from build123d import *

# Parameters (mm, degrees)
SKETCH_1_W           = 33.2
SKETCH_1_H           = 22
SKETCH_1_R           = 1.6
EXTRUDE_1_DEPTH      = 7
SKETCH_2_W           = 33.2
SKETCH_2_H           = 10.5
EXTRUDE_2_DEPTH      = 2
EXTRUDE_3_DEPTH      = 60
SKETCH_4_W           = 2
SKETCH_4_H           = 10.5
EXTRUDE_4_DEPTH      = 38.5
SKETCH_5_W           = 4
SKETCH_5_H           = 10.5
EXTRUDE_5_DEPTH      = 2
SKETCH_6_W           = 4
SKETCH_6_H           = 10.5
EXTRUDE_6_DEPTH      = 19.5
SKETCH_7_W           = 6
SKETCH_7_H           = 93.2
EXTRUDE_7_DEPTH      = 2
SKETCH_8_W           = 93.2
SKETCH_8_H           = 5
EXTRUDE_8_DEPTH      = 3
SKETCH_10_W          = 93.2
SKETCH_10_H          = 2
EXTRUDE_9_DEPTH      = 5.5
SKETCH_12_W          = 18
SKETCH_12_H          = 2
CUT_EXTRUDE_1_DEPTH  = 5.5
SKETCH_13_W          = 40
SKETCH_13_H          = 5
EXTRUDE_10_DEPTH     = 3.5
CUT_EXTRUDE_2_REACH  = 70.879
SKETCH_15_W          = 15.5
SKETCH_15_H          = 5
SKETCH_16_W          = 3.5
SKETCH_16_H          = 2.5
EXTRUDE_12_DEPTH     = 2
CUT_EXTRUDE_3_REACH  = 71.313
CHAMFER_1_SIZE       = 3.5
SKETCH_18_R          = 1.65
EXTRUDE_13_DEPTH     = 2
FILLET_1_R           = 2
SKETCH_19_W          = 4.5
SKETCH_19_H          = 21.5
CUT_EXTRUDE_4_DEPTH  = 5
CHAMFER_2_SIZE       = 3
CUT_EXTRUDE_5_REACH  = 74.561
SKETCH_20_R          = 1.65
EXTRUDE_14_REACH     = 73.895
SKETCH_21_R          = 4.5
SKETCH_21_R_2        = 1.65
EXTRUDE_15_DEPTH     = 6
EXTRUDE_16_DEPTH     = 4
CUT_EXTRUDE_6_REACH  = 83.84
SKETCH_24_R          = 1.65
CUT_EXTRUDE_7_REACH  = 84.171
SKETCH_26_W          = 2
SKETCH_26_H          = 10.5
CUT_EXTRUDE_8_DEPTH  = 5
SKETCH_27_W          = 2
SKETCH_27_H          = 2
EXTRUDE_17_DEPTH     = 10
CUT_EXTRUDE_9_DEPTH  = 2
CUT_EXTRUDE_10_REACH = 84.426
SKETCH_29_R          = 5.5
SKETCH_30_W          = 63
SKETCH_30_H          = 2
EXTRUDE_18_DEPTH     = 1


with BuildPart() as part:
    # 草图1 → 凸台-拉伸1 (new body)
    with BuildSketch(Plane(origin=(0, 0, 0), x_dir=(0, 0, -1), z_dir=(1, 0, 0))):
        with Locations((12.6, -4.5)):
            Rectangle(SKETCH_1_W, SKETCH_1_H)
        Circle(SKETCH_1_R, mode=Mode.SUBTRACT)
        with Locations((20, 0)):
            Circle(SKETCH_1_R, mode=Mode.SUBTRACT)
    extrude(amount=EXTRUDE_1_DEPTH)

    # 草图2 → 凸台-拉伸2 (add)
    with BuildSketch(Plane(origin=(7, 0, 0), x_dir=(0, 0, -1), z_dir=(1, 0, 0))):
        with Locations((12.6, 11.75)):
            Rectangle(SKETCH_2_W, SKETCH_2_H)
    extrude(amount=-EXTRUDE_2_DEPTH)

    # 草图3 → 凸台-拉伸3 (add)
    with BuildSketch(Plane.XY.offset(4)):
        Polygon((7, -15.5), (1, -15.5), (1, 4.5), (3, 4.5), (3, 6.5), (7, 6.5), align=None)
    extrude(amount=EXTRUDE_3_DEPTH)

    # 草图4 → 凸台-拉伸4 (add)
    with BuildSketch(Plane.XY.offset(4)):
        with Locations((6, 11.75)):
            Rectangle(SKETCH_4_W, SKETCH_4_H)
    extrude(amount=EXTRUDE_4_DEPTH)

    # 草图5 → 凸台-拉伸5 (add)
    with BuildSketch(Plane.XY.offset(42.5)):
        with Locations((5, 11.75)):
            Rectangle(SKETCH_5_W, SKETCH_5_H)
    extrude(amount=EXTRUDE_5_DEPTH)

    # 草图6 → 凸台-拉伸6 (add)
    with BuildSketch(Plane.XY.offset(44.5)):
        with Locations((5, 11.75)):
            Rectangle(SKETCH_6_W, SKETCH_6_H)
    extrude(amount=EXTRUDE_6_DEPTH)

    # 草图7 → 凸台-拉伸7 (add)
    with BuildSketch(Plane(origin=(0, 17, 0), x_dir=(1, 0, 0), z_dir=(0, 1, 0))):
        with Locations((4, -17.4)):
            Rectangle(SKETCH_7_W, SKETCH_7_H)
    extrude(amount=EXTRUDE_7_DEPTH)

    # 草图8 → 凸台-拉伸8 (add)
    with BuildSketch(Plane.ZY.offset(-1)):
        with Locations((17.4, 21.5)):
            Rectangle(SKETCH_8_W, SKETCH_8_H)
    extrude(amount=-EXTRUDE_8_DEPTH)

    # 草图10 → 凸台-拉伸9 (add)
    with BuildSketch(Plane.ZY.offset(-1)):
        with Locations((17.4, 23)):
            Rectangle(SKETCH_10_W, SKETCH_10_H)
    extrude(amount=EXTRUDE_9_DEPTH)

    # 草图12 → 切除-拉伸1 (cut)
    with BuildSketch(Plane.ZY.offset(4.5)):
        with Locations((-20.2, 23)):
            Rectangle(SKETCH_12_W, SKETCH_12_H)
    extrude(amount=-CUT_EXTRUDE_1_DEPTH, mode=Mode.SUBTRACT)

    # 草图13 → 凸台-拉伸10 (add)
    with BuildSketch(Plane.ZY.offset(-1)):
        with Locations((-9.2, 19.5)):
            Rectangle(SKETCH_13_W, SKETCH_13_H)
    extrude(amount=EXTRUDE_10_DEPTH)

    # 草图15 → 切除-拉伸2 (cut, up to next)
    with BuildSketch(Plane(origin=(4, 0, 0), x_dir=(0, 0, -1), z_dir=(1, 0, 0)), mode=Mode.PRIVATE) as cut_extrude_2_sk1:
        with Locations((21.45, 21.5)):
            Rectangle(SKETCH_15_W, SKETCH_15_H)
    cut_extrude_2_tool1 = extrude(cut_extrude_2_sk1.sketch, amount=-CUT_EXTRUDE_2_REACH, mode=Mode.PRIVATE) & part.part
    add(cut_extrude_2_tool1.solids().sort_by_distance((4, 21.5, -21.45))[0], mode=Mode.SUBTRACT)

    # 草图16 → 凸台-拉伸12 (add)
    with BuildSketch(Plane(origin=(0, 22, 0), x_dir=(1, 0, 0), z_dir=(0, 1, 0))):
        with Locations((-0.75, 12.45)):
            Rectangle(SKETCH_16_W, SKETCH_16_H)
    extrude(amount=EXTRUDE_12_DEPTH)

    # 草图17 → 切除-拉伸3 (cut, up to next)
    with BuildSketch(Plane(origin=(7, 0, 0), x_dir=(0, 0, -1), z_dir=(1, 0, 0)), mode=Mode.PRIVATE) as cut_extrude_3_sk1:
        Polygon((-47.5, 24), (-64, 8.613501079), (-64, 24), align=None)
    cut_extrude_3_tool1 = extrude(cut_extrude_3_sk1.sketch, amount=-CUT_EXTRUDE_3_REACH, mode=Mode.PRIVATE) & part.part
    add(cut_extrude_3_tool1.solids().sort_by_distance((7, 18.871167, 58.5))[0], mode=Mode.SUBTRACT)

    # 倒角1
    # the kernel refuses this chamfer: 3.5 mm, written as the material it takes off along each edge
    with BuildSketch(Plane(origin=(-4.5, 15.861407469, 56.227571974), x_dir=(0.9996219169112969, 0.020109211138415985, 0.018752142756900524), z_dir=(0, 0.6819983600625026, -0.7313537016191667))) as chamfer_1_piece_1:
        Polygon((CHAMFER_1_SIZE * 0.999621916911, CHAMFER_1_SIZE * 0.0274958766106), (-CHAMFER_1_SIZE * 0.0274958766106, CHAMFER_1_SIZE * 0.999621916911), (0, 0), align=None)
    extrude(amount=20.934339287, mode=Mode.SUBTRACT)

    # 草图18 → 凸台-拉伸13 (add)
    with BuildSketch(Plane.ZY.offset(2.5)):
        with BuildLine():
            Line((-11.337, 27.2), (-11.337, 24))
            Line((-11.337, 24), (-13.7, 24))
            Line((-13.7, 24), (-13.7, 19))
            Line((-13.7, 19), (-21.337, 19))
            Line((-21.337, 19), (-21.337, 27.2))
            ThreePointArc((-21.337, 27.2), (-16.337, 32.2), (-11.337, 27.2))
        make_face()
        with Locations((-16.337, 27.2)):
            Circle(SKETCH_18_R, mode=Mode.SUBTRACT)
    extrude(amount=-EXTRUDE_13_DEPTH)

    # 圆角1
    fillet_1_edges = [part.edges().sort_by_distance(p)[0] for p in [
        (-1.5, 24, -11.337),
        (-1.5, 19, -21.337),
    ]]
    fillet(fillet_1_edges, radius=FILLET_1_R)

    # 草图19 → 切除-拉伸4 (cut)
    with BuildSketch(Plane(origin=(0, 24, 0), x_dir=(1, 0, 0), z_dir=(0, 1, 0))):
        with Locations((1.75, 2.95)):
            Rectangle(SKETCH_19_W, SKETCH_19_H)
    extrude(amount=-CUT_EXTRUDE_4_DEPTH, mode=Mode.SUBTRACT)

    # 倒角2
    chamfer_2_edges = [part.edges().sort_by_distance(p)[0] for p in [
        (4, 24, 27.65),
        (1, 22, 30.22236871),
    ]]
    chamfer(chamfer_2_edges, length=CHAMFER_2_SIZE)

    # 草图20 → 切除-拉伸5 (cut, up to next)
    with BuildSketch(Plane(origin=(7, 0, 0), x_dir=(0, 0, -1), z_dir=(1, 0, 0)), mode=Mode.PRIVATE) as cut_extrude_5_sk1:
        with Locations((-62.5, 4)):
            Circle(SKETCH_20_R)
    cut_extrude_5_tool1 = extrude(cut_extrude_5_sk1.sketch, amount=-CUT_EXTRUDE_5_REACH, mode=Mode.PRIVATE) & part.part
    add(cut_extrude_5_tool1.solids().sort_by_distance((7, 4, 62.5))[0], mode=Mode.SUBTRACT)

    # 凸台-拉伸14: up to this face of the body (flat: up to its plane)
    extrude_14_end = Plane(part.part.faces().sort_by_distance((7, 1.498387626, 16.627822956))[0])
    # 草图21 → 凸台-拉伸14 (add, up to the picked face)
    with BuildSketch(Plane.ZY.offset(-1), mode=Mode.PRIVATE) as extrude_14_sk1:
        with Locations((62.5, 4)):
            Circle(SKETCH_21_R)
        with Locations(Location((62.5, 4, 0), (0, 0, 180))):
            Circle(SKETCH_21_R_2, mode=Mode.SUBTRACT)
    extrude_14_tool1 = split(extrude(extrude_14_sk1.sketch, amount=-EXTRUDE_14_REACH, mode=Mode.PRIVATE), bisect_by=extrude_14_end, keep=Keep.BOTH, mode=Mode.PRIVATE)
    add(extrude_14_tool1.solids().sort_by(Axis((1, 4, 58.127279), (1, 0, 0)))[0])

    # 草图22 → 凸台-拉伸15 (add)
    with BuildSketch(Plane.ZY.offset(-1)):
        with BuildLine():
            Line((66.198595209, 6.563277878), (75, -1.644164869))
            Line((75, -1.644164869), (75, -15.5))
            Line((75, -15.5), (64, -15.5))
            Line((64, -15.5), (64, -0.242640687))
            ThreePointArc((64, -0.242640687), (66.782111619, 2.616699568), (66.198595209, 6.563277878))
        make_face()
    extrude(amount=-EXTRUDE_15_DEPTH)

    # 草图23 → 凸台-拉伸16 (add)
    with BuildSketch(Plane(origin=(7, 0, 0), x_dir=(0, 0, -1), z_dir=(1, 0, 0))):
        Polygon((-64, 8.613501079), (-64.799032902, 7.868390843), (-64, 8.242640687), align=None)
    extrude(amount=-EXTRUDE_16_DEPTH)

    # 草图24 → 切除-拉伸6 (cut, up to next)
    with BuildSketch(Plane.ZY.offset(-1), mode=Mode.PRIVATE) as cut_extrude_6_sk1:
        with Locations(Location((71, -10.5, 0), (0, 0, 270))):
            Circle(SKETCH_24_R)
    cut_extrude_6_tool1 = extrude(cut_extrude_6_sk1.sketch, amount=-CUT_EXTRUDE_6_REACH, mode=Mode.PRIVATE) & part.part
    add(cut_extrude_6_tool1.solids().sort_by_distance((1, -10.5, 71))[0], mode=Mode.SUBTRACT)

    # 草图25 → 切除-拉伸7 (cut, up to next)
    with BuildSketch(Plane.ZY.offset(-5), mode=Mode.PRIVATE) as cut_extrude_7_sk1:
        with BuildLine():
            Line((17.8, 8), (-14.2, 8))
            ThreePointArc((-14.2, 8), (-17.95, 11.75), (-14.2, 15.5))
            Line((-14.2, 15.5), (17.8, 15.5))
            ThreePointArc((17.8, 15.5), (21.55, 11.75), (17.8, 8))
        make_face()
    cut_extrude_7_tool1 = extrude(cut_extrude_7_sk1.sketch, amount=-CUT_EXTRUDE_7_REACH, mode=Mode.PRIVATE) & part.part
    add(cut_extrude_7_tool1.solids().sort_by_distance((5, 11.75, 1.8))[0], mode=Mode.SUBTRACT)

    # 草图26 → 切除-拉伸8 (cut)
    with BuildSketch(Plane(origin=(0, 0, 42.5), x_dir=(-1, 0, 0), z_dir=(0, 0, -1))):
        with Locations((-4, 11.75)):
            Rectangle(SKETCH_26_W, SKETCH_26_H)
    extrude(amount=-CUT_EXTRUDE_8_DEPTH, mode=Mode.SUBTRACT)

    # 草图27 → 凸台-拉伸17 (add)
    with BuildSketch(Plane.XY.offset(4)):
        with Locations((2, 5.5)):
            Rectangle(SKETCH_27_W, SKETCH_27_H)
    extrude(amount=EXTRUDE_17_DEPTH)

    # 草图28 → 切除-拉伸9 (cut)
    with BuildSketch(Plane.ZY.offset(-1)):
        Polygon((67, 0.394553878), (67, -15.5), (75, -15.5), (75, -1.644164869), (69.70409784, 3.29434379), align=None)
    extrude(amount=-CUT_EXTRUDE_9_DEPTH, mode=Mode.SUBTRACT)

    # 草图29 → 切除-拉伸10 (cut, up to next)
    with BuildSketch(Plane(origin=(7, 0, 0), x_dir=(0, 0, -1), z_dir=(1, 0, 0)), mode=Mode.PRIVATE) as cut_extrude_10_sk1:
        with Locations((34, 3.1)):
            Circle(SKETCH_29_R)
    cut_extrude_10_tool1 = extrude(cut_extrude_10_sk1.sketch, amount=-CUT_EXTRUDE_10_REACH, mode=Mode.PRIVATE) & part.part
    add(cut_extrude_10_tool1.solids().sort_by_distance((7, 3.1, -34))[0], mode=Mode.SUBTRACT)

    # 草图30 → 凸台-拉伸18 (add)
    with BuildSketch(Plane.ZY.offset(-1)):
        with Locations((35.5, -5.5)):
            Rectangle(SKETCH_30_W, SKETCH_30_H)
    extrude(amount=EXTRUDE_18_DEPTH)


solid = part.part
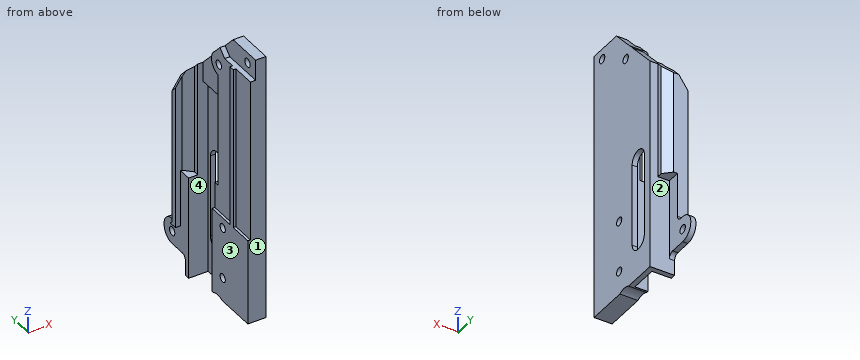
Part model, mm, in its own coordinate system. Face numbers are marked on the shaded views. A direction names the side the tool comes from. Give positions to 0.01 mm unless a question says otherwise; leave off trailing zeros. Order: outer loops, then holes, each group sorted by start corner. A loop starts at its lowest first (then second) coordinate and runs counter-clockwise, first axis right, second up. Notation, with made-up numbers: (65, 32) - (100, 32) arc R18 cw to (100, 67) - close; hole circle Ø11 at (64, -25.5). An arc over 180 degrees is marked (long way). Use a Markdown table: item, result.
1) Saw through at C-C on y = -3. List the corners of the cut face in (x, z), plus the area to 3 significant figures.
Checked values:
| item | result |
|---|---|
| outline | (0, -29.2) - (7, -29.2) - (7, 75) - (3, 75) - (3, 67) - (1, 67) - (1, 4) - (0, 4) - close |
| area | 642 mm² |
2) Saw through at D-D on x = -3.5. List the corners of the cut face in (y, z).
Checked values:
| item | result |
|---|---|
| outline | (22, -11.2) - (25.27, -11.2) arc R2 cw to (24, -9.34) - (24, 43.83) - (22, 45.98) - close |
3) Flat gauge pins, fed straight in: P1, Ø6, axis at x = 1, y = 22.5, coming from the -Z side; P2, Ø4, axis at y = 9.5, z = 62.5, coming from the -X side; P3, Ø1.1, axis at x = 0.5, y = -12, coming from the +Z side. Where does each tip first touch, or does it go through?
Checked values:
| item | result |
|---|---|
| P1 | z = -21.67 |
| P2 | x = 1 |
| P3 | z = 67 |
4) Probe L1, parallel to Y at x = 3, z = -20; L2, parallel to Y at x = 4.25, z = -11; L3, parallel to Z at x = 5.2, y = -10.5. List the from-to ranges inside material, lowest first. Write a range as from..to.
Checked values:
| item | result |
|---|---|
| L1 | -15.5..-1.6, 1.6..6.5, 17..19 |
| L2 | -15.5..6.5, 17..19 |
| L3 | -29.2..69.35, 72.65..75 |
5) Saw through at B-B on z = 71. List the corners of the cut face in (x, y), plus the area to 3 significant figures.
Checked values:
| item | result |
|---|---|
| outline | (3, -15.5) - (7, -15.5) - (7, -12.15) - (3, -12.15) - close; (3, -8.85) - (7, -8.85) - (7, 2.09) - (3, 2.09) - close |
| area | 57.1 mm² |
6) 3-axis set-ups, long thin cutter, end or side, ignore diameter. For the marked faces 1, 2, 3 and 4: which of +Z, -Z, +X, -X, +Y, -Y reach the whole face in a straight line?
Checked values:
| item | result |
|---|---|
| face 1 | +Z, -Z, +X, -X, -Y |
| face 2 | -Z, +X, +Y |
| face 3 | +Z, -Z, -X, -Y |
| face 4 | -Z, -X |
7) Saw through at A-A on y = -10.5. List the corners of the cut face in (x, z).
Checked values:
| item | result |
|---|---|
| outline | (0, -29.2) - (7, -29.2) - (7, 69.35) - (3, 69.35) - (3, 67) - (1, 67) - (1, 4) - (0, 4) - close; (3, 72.65) - (7, 72.65) - (7, 75) - (3, 75) - close |
